Part model, mm, in its own coordinate system. A direction names the side the tool comes from. Give positions to 0.01 mm unless a question says otherwise; leave off trailing zeros. Loops run counter-clockwise (first coordinate to the right, second up) from the corner with the lowest first, then second, coordinate; pieces in that order, holes last. Notation, with made-up numbers: M 58.5,-31 L 113.5,-31 A33 cw 113.5,8 Z; hole C 25,-16 d11. An arc over 180 degrees is marked long. Put each result on its own line as item: value. Start each with the question number.
```python
from build123d import *

# Parameters (mm, degrees)
F0_W     = 12
F0_H     = 12
F1_DEPTH = 40


with BuildPart() as f1:
    # F0 (on Top) → F1 (new body)
    with BuildSketch(Plane.XY):
        with BuildLine():
            ThreePointArc((-18.337186, 24.095786), (-16.687389, 23.478766), (-15.016882, 22.920239))
            ThreePointArc((-15.016882, 22.920239), (-16.656306, 23.56656), (-18.337186, 24.095786))
        make_face()
        with BuildLine():
            ThreePointArc((15.016882, 22.920239), (0, 20.611887), (-15.016882, 22.920239))
            ThreePointArc((-15.016882, 22.920239), (-16.687389, 23.478766), (-18.337186, 24.095786))
            ThreePointArc((-18.337186, 24.095786), (-50, 0), (-18.337186, -24.095786))
            ThreePointArc((-18.337186, -24.095786), (-16.687389, -23.478766), (-15.016882, -22.920239))
            ThreePointArc((-15.016882, -22.920239), (0, -20.611887), (15.016882, -22.920239))
            ThreePointArc((15.016882, -22.920239), (16.687389, -23.478766), (18.337186, -24.095786))
            ThreePointArc((18.337186, -24.095786), (50, 0), (18.337186, 24.095786))
            ThreePointArc((18.337186, 24.095786), (16.687389, 23.478766), (15.016882, 22.920239))
        make_face()
        with BuildLine():
            ThreePointArc((-13, -11.324752), (-41.5, 0), (-13, 11.324752))
            Line((-13, 11.324752), (-13, -11.324752))
        make_face(mode=Mode.SUBTRACT)
        Rectangle(F0_W, F0_H, mode=Mode.SUBTRACT)
        with BuildLine():
            Line((13, -11.324752), (13, 11.324752))
            ThreePointArc((13, 11.324752), (41.5, 0), (13, -11.324752))
        make_face(mode=Mode.SUBTRACT)
        with BuildLine():
            ThreePointArc((18.337186, 24.095786), (16.656306, 23.56656), (15.016882, 22.920239))
            ThreePointArc((15.016882, 22.920239), (16.687389, 23.478766), (18.337186, 24.095786))
        make_face()
        with BuildLine():
            ThreePointArc((-15.016882, -22.920239), (-16.687389, -23.478766), (-18.337186, -24.095786))
            ThreePointArc((-18.337186, -24.095786), (-16.656306, -23.56656), (-15.016882, -22.920239))
        make_face()
        with BuildLine():
            ThreePointArc((15.016882, -22.920239), (16.656306, -23.56656), (18.337186, -24.095786))
            ThreePointArc((18.337186, -24.095786), (16.687389, -23.478766), (15.016882, -22.920239))
        make_face()
    extrude(amount=F1_DEPTH)


solid = f1.part
```
1) Mould opens along X. For faces 1 (the cylindrical face through (16.68, 23.575, 19.72)), 2 (the flat face through (10, 0, 40)) say: +X half, -X half, draft (parallel to the pull), parting line (faces both ways), or undercut.
2) Wall check: L1, parallel to X at y = 10, z = 9.5; L2, parallel to Y at x = -25, z = 15.5; L3, parallel to X at y = -10.5, z = 38.5. Give the ranges that are in metal, low to high.
3) Band-saw the part on C-C on z = 29.5. Give the cut face in (x, y).
4) Pin check, flat tips, straight feed: pin 1 Ø5 at (x, z) = (37, 7) entering from -Y; pin 2 Ø8 at (y, z) = (-19, 18) entering from +X; pin 3 Ø6 at (x, z) = (-34.5, 17) entering from +Y. Stop position of each tip, or through.
5) Which spindle directions (+Z, -Z, +X, -X, +Y, -Y) get a long thin tool onto all of the face, cutting with end or side? Do faces 3 (the flat face through (10, 0, 0)), 4 (the cylindrical face through (16.633, -23.558, 19.72)), 5 (the flat face through (-6, 0, 20)), 6 (the cylindrical face through (-16.633, 23.558, 19.72)). Say none if no direction does.
6) Band-saw the part on B-B on y = 0. Give the cut face in (x, z), then the cut area to 3 significant figures.
7) Band-saw the part on D-D on x = 10.5. Give the cut face in (y, z).
8) Band-saw the part on A-A on x = -25. Give the cut face in (y, z), then the cut area to 3 significant figures.
Evaluation:
1. face 1: undercut
1. face 2: draft
2. L1: -47.91 to -38.12, -13 to 13, 38.12 to 47.91
2. L2: -25 to -16.5, 16.5 to 25
2. L3: -47.69 to -37.73, -13 to 13, 37.73 to 47.69
3. outline: M -18.34,-24.1 A25 ccw -15.02,-22.92 A50 cw 15.02,-22.92 A25 ccw 18.34,-24.1 A25 ccw long 18.34,24.1 A25 ccw 15.02,22.92 A50 cw -15.02,22.92 A25 ccw -18.34,24.1 A25 ccw long Z; hole M -13,-11.32 L -13,11.32 A16.5 ccw long Z; hole M -6,-6 L 6,-6 L 6,6 L -6,6 Z; hole M 13,-11.32 A16.5 ccw long 13,11.32 Z
4. pin 1: y = -23.12
4. pin 2: x = 45
4. pin 3: y = 24.14
5. face 3: -Z, +X, -X, +Y, -Y
5. face 4: +Z, -Z, -Y
5. face 5: +Z, -Z
5. face 6: +Z, -Z, +Y
6. outline: M -50,0 L -41.5,0 L -41.5,40 L -50,40 Z; M -13,0 L -6,0 L -6,40 L -13,40 Z; M 6,0 L 13,0 L 13,40 L 6,40 Z; M 41.5,0 L 50,0 L 50,40 L 41.5,40 Z
6. area: 1,240 mm2
7. outline: M -21.73,0 L 21.73,0 L 21.73,40 L -21.73,40 Z
8. outline: M -25,0 L -16.5,0 L -16.5,40 L -25,40 Z; M 16.5,0 L 25,0 L 25,40 L 16.5,40 Z
8. area: 680 mm2
